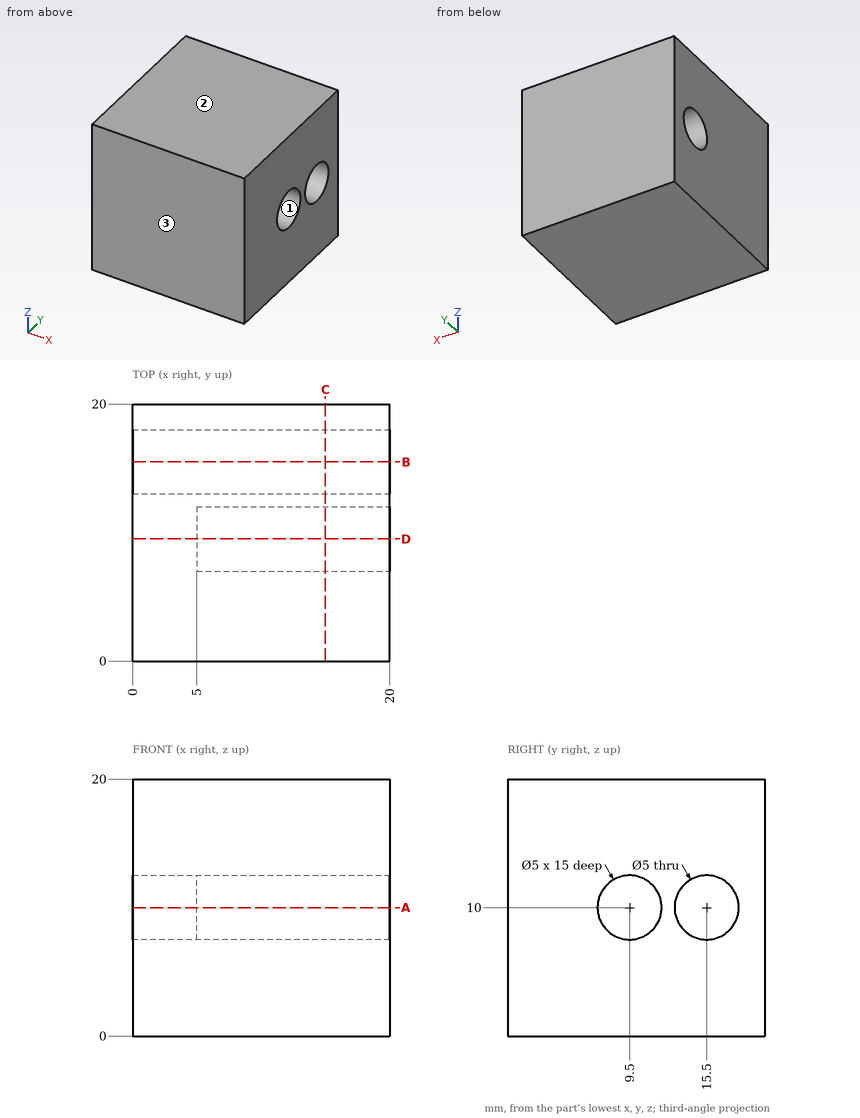
Part print with two shaded views. Sizes in mm from the minimum x, y, z corner. Round coordinates to 2 decimals unless told otherwise and drop trailing zeros. Write each loop counter-clockwise with the first axis right and the second up, starting at its lowest first coordinate (ties: lowest second). Pieces come first, ordered by that corner, then holes. Notation, with made-up numbers: M 46.5,9 L 58.5,9 A21 ccw 58.5,35 Z; hole C 51,57 d6. An arc over 180 degrees is marked long. Answer as CSV lines item,"result". Start each with the question number.
1) Band-saw the part on C-C (x = 15). List the corners of the cut face in (y, z).
2) Drill centre lines: L1, parallel to Y at x = 14, z = 10; L2, parallel to X at y = 9.5, z = 11.25; L3, parallel to Y at x = 15.5, z = 8. Where is each one in solid material? Low to high.
3) Band-saw the part on A-A (z = 10). List the corners of the cut face in (x, y), then the cut area to 3 significant figures.
4) Mould opens along Z. For the marked faces 1, 2 and 3 say: +Z half, -Z half, draft (parallel to the pull), parting line (faces both ways), or undercut.
5) Band-saw the part on B-B (y = 15.5). List the corners of the cut face in (x, z), then the cut area to 3 significant figures.
6) Band-saw the part on D-D (y = 9.5). List the corners of the cut face in (x, z), then the cut area to 3 significant figures.
7) Drop a flat-ended pin along its axis: pin 1 (6 mm diameter, centred on y = 13, z = 8, fed in from -X). Give the stop position or say it passes through.
Worked out:
1,outline,"M 0,0 L 20,0 L 20,20 L 0,20 Z; hole C 9.5,10 d5; hole C 15.5,10 d5"
2,L1,"0 to 7, 12 to 13, 18 to 20"
2,L2,"0 to 5"
2,L3,"0 to 8, 11 to 14, 17 to 20"
3,outline,"M 0,0 L 20,0 L 20,7 L 5,7 L 5,12 L 20,12 L 20,13 L 0,13 Z; M 0,18 L 20,18 L 20,20 L 0,20 Z"
3,area,"225 mm²"
4,face 1,"undercut"
4,face 2,"+Z half"
4,face 3,"draft"
5,outline,"M 0,0 L 20,0 L 20,7.5 L 0,7.5 Z; M 0,12.5 L 20,12.5 L 20,20 L 0,20 Z"
5,area,"300 mm²"
6,outline,"M 0,0 L 20,0 L 20,7.5 L 5,7.5 L 5,12.5 L 20,12.5 L 20,20 L 0,20 Z"
6,area,"325 mm²"
7,pin 1,"x = 0"
